```python
from build123d import *

# Parameters (mm, degrees)
SKETCH1_W           = 150
SKETCH1_H           = 140
SKETCH1_R           = 2.85
SKETCH1_R_2         = 1.75
SKETCH1_W_2         = 80
SKETCH1_H_2         = 51
BOSS_EXTRUDE1_DEPTH = 5
SKETCH2_W           = 100
SKETCH2_H           = 71
SKETCH2_W_2         = 80
SKETCH2_H_2         = 51
CUT_EXTRUDE1_DEPTH  = 3


with BuildPart() as part:
    # Sketch1 → Boss-Extrude1 (new body)
    with BuildSketch(Plane.XY):
        with Locations((3.078431373, -11.336177597)):
            Rectangle(SKETCH1_W, SKETCH1_H)
        with Locations((70.078431373, -73.336177597)):
            Circle(SKETCH1_R, mode=Mode.SUBTRACT)
        with Locations((-63.921568627, -73.336177597)):
            Circle(SKETCH1_R, mode=Mode.SUBTRACT)
        with Locations((-63.921568627, 50.663822403)):
            Circle(SKETCH1_R, mode=Mode.SUBTRACT)
        with Locations((70.078431373, 50.663822403)):
            Circle(SKETCH1_R, mode=Mode.SUBTRACT)
        with Locations((-34.421568627, 13.963822403)):
            Circle(SKETCH1_R_2, mode=Mode.SUBTRACT)
        with Locations((23.578431373, 13.963822403)):
            Circle(SKETCH1_R_2, mode=Mode.SUBTRACT)
        with Locations((3.078431373, -13.836177597)):
            Rectangle(SKETCH1_W_2, SKETCH1_H_2, mode=Mode.SUBTRACT)
    extrude(amount=BOSS_EXTRUDE1_DEPTH)

    # Sketch2 → Cut-Extrude1 (cut)
    with BuildSketch(Plane(origin=(0, 0, 0), x_dir=(-1, 0, 0), z_dir=(0, 0, -1))):
        with Locations((-3.078431373, -13.836177597)):
            Rectangle(SKETCH2_W, SKETCH2_H)
        with Locations((-3.078431373, -13.836177597)):
            Rectangle(SKETCH2_W_2, SKETCH2_H_2, mode=Mode.SUBTRACT)
    extrude(amount=-CUT_EXTRUDE1_DEPTH, mode=Mode.SUBTRACT)


solid = part.part
```
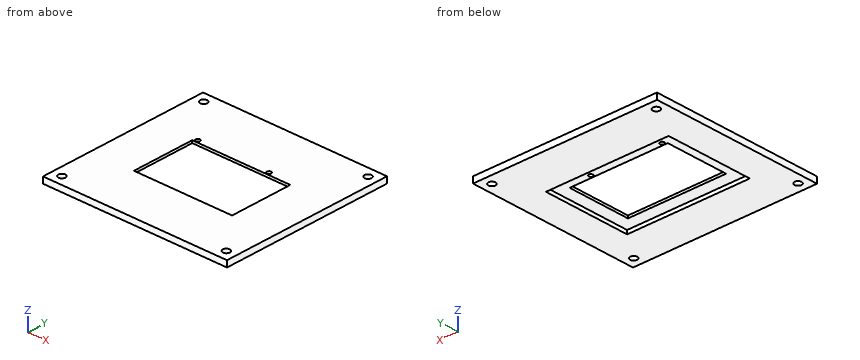
Check sheet for the modelled part. Datum: model origin and axes. Units: mm. Round coordinates to 2 decimals unless told otherwise and drop trailing zeros. Order: outer loops, then holes, each group sorted by start corner. A loop starts at its lowest first (then second) coordinate and runs counter-clockwise, first axis right, second up. Notation, with made-up numbers: (51, 32.25) -> (77, 32.25) arc R20 cw to (77, 56.25) -> close; hole circle Ø6 at (80.25, 77). An arc over 180 degrees is marked (long way). One line per item, written item: value. Start each with the question number.
Q1. Cross-section at C-C (y = -47.5). Record the boundary of the cut face in (x, z), and give its area (3 significant figures).
Q2. Cross-section at D-D (z = 1.8). Record the boundary of the cut face in (x, y), and give its area (3 significant figures).
Q3. Cross-section at A-A (x = -23.5). Record the boundary of the cut face in (y, z), and give its area (3 significant figures).
Q4. Cross-section at B-B (y = -24.5). Record the boundary of the cut face in (x, z).
Q5. Thickness scan on line 1 (X direction, y = -73.5, z = 2.1); line 2 (X direction, y = 5.5, z = 4.35); line 3 (Y direction, x = 51, z = 2). Record the ranges inside material, lowest first.
Q6. Gauge pin test, flat end, axial feed: pin 1 Ø4 at (x, y) = (-34.42, 13.96) entering from -Z. Record the tip position at first contact, or that the pin passes through.
Completed:
1. outline: (-71.92, 0) -> (-46.92, 0) -> (-46.92, 3) -> (53.08, 3) -> (53.08, 0) -> (78.08, 0) -> (78.08, 5) -> (-71.92, 5) -> close
1. area: 450 mm²
2. outline: (-71.92, -81.34) -> (78.08, -81.34) -> (78.08, 58.66) -> (-71.92, 58.66) -> close; hole circle Ø5.7 at (-63.92, -73.34); hole circle Ø5.7 at (-63.92, 50.66); hole (-46.92, -49.34) -> (53.08, -49.34) -> (53.08, 21.66) -> (-46.92, 21.66) -> close; hole circle Ø5.7 at (70.08, -73.34); hole circle Ø5.7 at (70.08, 50.66)
2. area: 13,800 mm²
3. outline: (-81.34, 0) -> (-49.34, 0) -> (-49.34, 3) -> (-39.34, 3) -> (-39.34, 5) -> (-81.34, 5) -> close; (11.66, 3) -> (21.66, 3) -> (21.66, 0) -> (58.66, 0) -> (58.66, 5) -> (11.66, 5) -> close
3. area: 385 mm²
4. outline: (-71.92, 0) -> (-46.92, 0) -> (-46.92, 3) -> (-36.92, 3) -> (-36.92, 5) -> (-71.92, 5) -> close; (43.08, 3) -> (53.08, 3) -> (53.08, 0) -> (78.08, 0) -> (78.08, 5) -> (43.08, 5) -> close
5. line 1: x = -71.92 to -66.77, -61.08 to 67.23, 72.92 to 78.08
5. line 2: x = -71.92 to -36.92, 43.08 to 78.08
5. line 3: y = -81.34 to -49.34, 21.66 to 58.66
6. pin 1: stops at z = 3
